from build123d import *

# Parameters (mm, degrees)
PAD_DEPTH       = 215
POCKET_DEPTH    = 104.001
SKETCH003_W     = 65
SKETCH003_H     = 110
PAD002_DEPTH    = 22
PAD003_DEPTH    = 18
PAD004_DEPTH    = 23
POCKET001_DEPTH = 79.001


with BuildPart() as part:
    # Sketch → Pad (new body)
    with BuildSketch(Plane.XY):
        with BuildLine():
            Line((-54, 95), (-54, 0))
            Line((-54, 0), (-50, 0))
            Line((-50, 0), (-50, -61))
            ThreePointArc((-50, -61), (-49.4142135624, -62.4142135624), (-48, -63))
            Line((-48, -63), (-23.5, -63))
            ThreePointArc((-23.5, -63), (-22.0857864376, -62.4142135624), (-21.5, -61))
            Line((-21.5, -61), (-21.5, -27.5))
            ThreePointArc((-14.5, -20.5), (-19.4497474683, -22.5502525317), (-21.5, -27.5))
            Line((-14.5, -20.5), (28.5, -20.5))
            ThreePointArc((35.5, -27.5), (33.4497474683, -22.5502525317), (28.5, -20.5))
            Line((35.5, -27.5), (35.5, -61))
            ThreePointArc((35.5, -61), (36.0857864376, -62.4142135624), (37.5, -63))
            Line((37.5, -63), (48, -63))
            ThreePointArc((48, -63), (49.4142135624, -62.4142135624), (50, -61))
            Line((50, -61), (50, 0))
            Line((50, 0), (54, 0))
            Line((54, 0), (54, 95))
            ThreePointArc((54, 95), (53.4142135624, 96.4142135624), (52, 97))
            Line((52, 97), (-52, 97))
            ThreePointArc((-52, 97), (-53.4142135624, 96.4142135624), (-54, 95))
        make_face()
    extrude(amount=PAD_DEPTH)

    # Sketch001 (on DatumPlane) → Pocket (cut, through all)
    with BuildSketch(Plane.YZ.offset(50)):
        with BuildLine():
            Line((-20.5, 220), (-20.5, 97.5))
            ThreePointArc((-63, 55), (-32.9479617996, 67.4479617996), (-20.5, 97.5))
            Line((-63, 55), (-68, 55))
            Line((-68, 55), (-68, 220))
            Line((-68, 220), (-20.5, 220))
        make_face()
    extrude(amount=-POCKET_DEPTH, mode=Mode.SUBTRACT)

    # Sketch003 (on DatumPlane) → Pad002 (join)
    with BuildSketch(Plane.XZ):
        with Locations((7, 163)):
            Rectangle(SKETCH003_W, SKETCH003_H)
    extrude(amount=PAD002_DEPTH)

    # Sketch004 (on DatumPlane) → Pad003 (join, symmetric)
    with BuildSketch(Plane.YZ.offset(7)):
        Polygon((-22, 218), (-60.7693471681, 168.301532014), (-45, 156), (-22, 156), align=None)
    extrude(amount=PAD003_DEPTH, both=True)

    # Sketch005 (on DatumPlane) → Pad004 (join)
    with BuildSketch(Plane.XZ.offset(22)):
        Polygon((13, 136), (1, 136), (-11, 151), (-11, 156), (25, 156), (25, 151), align=None)
    extrude(amount=PAD004_DEPTH)

    # Sketch007 (on DatumPlane) → Pocket001 (cut, through all)
    with BuildSketch(Plane.YZ.offset(25)):
        Polygon((-45, 151), (-38, 136), (-35, 136), (-22, 146), (-22, 135), (-46, 135), (-46, 151), align=None)
    extrude(amount=-POCKET001_DEPTH, mode=Mode.SUBTRACT)


solid = part.part
Geometry check sheet. Reference: the model listing, model coordinates, mm. A direction names the side the tool comes from. Give positions to 0.01 mm unless a question says otherwise; leave off trailing zeros. Order: outer loops, then holes, each group sorted by start corner. A loop starts at its lowest first (then second) coordinate and runs counter-clockwise, first axis right, second up. Notation, with made-up numbers: (62, 33) - (66, 33) arc R23 cw to (66, 42) - close; hole circle Ø11 at (21, -1.5). An arc over 180 degrees is marked (long way). Use one line per item in the form item = value.
1) Sectioned sample at D-D (z = 103). Record the boundary of the cut face in (x, y), and give its area (3 significant figures).
Working result:
outline = (-54, 0) - (-50, 0) - (-50, -20.5) - (50, -20.5) - (50, 0) - (54, 0) - (54, 95) arc R2 ccw to (52, 97) - (-52, 97) arc R2 ccw to (-54, 95) - close
area = 12,500 mm^2
2) Sectioned sample at B-B (x = 6). Record the boundary of the cut face in (y, z), and give its area (3 significant figures).
Working result:
outline = (-60.77, 168.3) - (-45, 156) - (-45, 151) - (-38, 136) - (-35, 136) - (-22, 146) - (-22, 108) - (-20.5, 108) - (-20.5, 0) - (97, 0) - (97, 215) - (0, 215) - (0, 218) - (-22, 218) - close
area = 27,200 mm^2
3) Depth check by flat-ended pin: pin 1 Ø2.5 at (x, z) = (7.5, 154) entering from -Y; pin 2 Ø1.2 at (x, z) = (51.5, 120.5) entering from -Y; pin 3 Ø19.5 at (y, z) = (-42, 180) entering from +X. Enter the tip coordinate at first touch or a pass-through.
Working result:
pin_1 = -45
pin_2 = 0
pin_3 = 25
4) Access from +Z, -Z, +X, -X, +Y, -Y to the whole of each face (thin tool, end or side, straight path). Record for faces 4 (the face through (7, -45, 154)), 5 (the face through (25, -37, 178)), 6 (the face through (-19.4, -22.5, 37.2)), 7 (the face through (-11, -37, 177)).
Working result:
face_4 = -Z, +X, -X, -Y
face_5 = +Z, -Z, +X, -Y
face_6 = -Z, -Y
face_7 = +Z, -Z, -X, -Y
5) Sectioned sample at A-A (z = 140). Record the boundary of the cut face in (x, y).
Working result:
outline = (-54, 0) - (-50, 0) - (-50, -20.5) - (-25.5, -20.5) - (-25.5, -22) - (39.5, -22) - (39.5, -20.5) - (50, -20.5) - (50, 0) - (54, 0) - (54, 95) arc R2 ccw to (52, 97) - (-52, 97) arc R2 ccw to (-54, 95) - close; (-2.2, -39.87) - (16.2, -39.87) - (16.2, -29.8) - (-2.2, -29.8) - close
6) Material ranges on probe 1 along Z at (x, y) = (-46, 80.5); probe 2 along Z at (x, y) = (47, -27.5); probe 3 along Y at (x, z) = (-18, 121), recorded low to high. Write a range as from..to.
Working result:
probe_1 = 0..215
probe_2 = 0..74.13
probe_3 = -22..97
7) Sectioned sample at C-C (z = 31). Record the boundary of the cut face in (x, y).
Working result:
outline = (-54, 0) - (-50, 0) - (-50, -61) arc R2 ccw to (-48, -63) - (-23.5, -63) arc R2 ccw to (-21.5, -61) - (-21.5, -27.5) arc R7 cw to (-14.5, -20.5) - (28.5, -20.5) arc R7 cw to (35.5, -27.5) - (35.5, -61) arc R2 ccw to (37.5, -63) - (48, -63) arc R2 ccw to (50, -61) - (50, 0) - (54, 0) - (54, 95) arc R2 ccw to (52, 97) - (-52, 97) arc R2 ccw to (-54, 95) - close
8) Draft check along X on faces 1 (the face through (-6.25, -33.34, 145.06)), 2 (the face through (-21.5, -44, 28)), 3 (the face through (7, -22, 139)). Enter one of: released by +X, released by -X, zero draft, split by the parting line, or undercut.
Working result:
face_1 = released by -X
face_2 = undercut
face_3 = zero draft
